from build123d import *

# Parameters (mm, degrees)
F2_DEPTH = 1.2
F3_DEPTH = 2.4
F4_R     = 2
F5_R     = 1
F6_SIZE  = 0.4


with BuildPart() as f2:
    # F1 (on Top) → F2 (new body)
    with BuildSketch(Plane.XY):
        Polygon((-15.6, 7.5), (-15.6, 5.7), (-0.9, 0), (-15.6, -5.7), (-15.6, -7.5), (-0.6, -7.5), (-0.6, 0), (-0.6, 7.5), align=None)
    extrude(amount=F2_DEPTH)



with BuildPart() as f2b:
    # F1 (on Top) → F2, piece 2 (new body)
    with BuildSketch(Plane.XY):
        Polygon((0.9, 0), (15.6, 5.7), (15.6, 7.5), (0.6, 7.5), (0.6, 0), (0.6, -7.5), (15.6, -7.5), (15.6, -5.7), align=None)
    extrude(amount=F2_DEPTH)


with BuildPart() as f2_1:
    add(f2.part)

    add(f2b.part)  # F3 merges F2b
    # F1 (on Top) → F3 (join)
    with BuildSketch(Plane.XY):
        Polygon((0, 8.7), (-16.8, 8.7), (-16.8, 5.7), (-15.6, 5.7), (-15.6, 7.5), (-0.6, 7.5), (-0.6, 0), (-0.6, -7.5), (-15.6, -7.5), (-15.6, -5.7), (-16.8, -5.7), (-16.8, -8.7), (0, -8.7), (16.8, -8.7), (16.8, -5.7), (15.6, -5.7), (15.6, -7.5), (0.6, -7.5), (0.6, 0), (0.6, 7.5), (15.6, 7.5), (15.6, 5.7), (16.8, 5.7), (16.8, 8.7), align=None)
    extrude(amount=F3_DEPTH)

    # F4
    f4_edges = [f2_1.edges().sort_by_distance(p)[0] for p in [
        (-0.9, 0, 0.6),
        (0.9, 0, 0.6),
    ]]
    fillet(f4_edges, radius=F4_R)

    # F5
    f5_edges = [f2_1.edges().sort_by_distance(p)[0] for p in [
        (16.8, -8.7, 1.2),
        (16.8, 8.7, 1.2),
        (-16.8, -8.7, 1.2),
        (-16.8, 8.7, 1.2),
    ]]
    fillet(f5_edges, radius=F5_R)

    # F6
    f6_edges = [f2_1.edges().sort_by_distance(p)[0] for p in [
        (16.8, 6.7, 0),
        (16.507107, 8.407107, 0),
        (16.2, 5.7, 0),
        (0, 8.7, 0),
        (10.654511, 3.782361, 0),
        (-16.507107, 8.407107, 0),
        (4.432077, 0, 0),
        (-16.8, 6.7, 0),
        (10.654511, -3.782361, 0),
        (-16.2, 5.7, 0),
        (16.2, -5.7, 0),
        (-10.654511, 3.782361, 0),
        (16.8, -6.7, 0),
        (-4.432077, 0, 0),
        (16.507107, -8.407107, 0),
        (-10.654511, -3.782361, 0),
        (0, -8.7, 0),
        (-16.2, -5.7, 0),
        (-16.507107, -8.407107, 0),
        (-16.8, -6.7, 0),
        (-10.654511, -3.782361, 1.2),
        (4.432077, 0, 1.2),
    ]]
    chamfer(f6_edges, length=F6_SIZE)


solid = f2_1.part
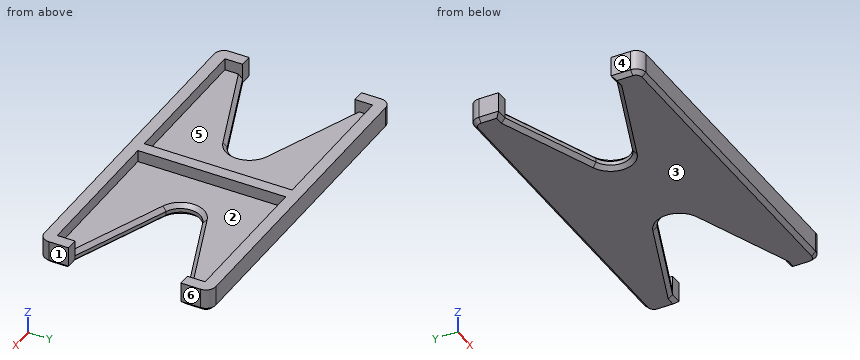
Read the model definition and answer for the solid it produces. Units are mm, in the model's axes. Face numbers are marked on the shaded views. A direction names the side the tool comes from. Coordinates: 2 decimals unless noted, no trailing zeros. Loops run counter-clockwise (first coordinate to the right, second up) from the corner with the lowest first, then second, coordinate; pieces in that order, holes last.
Q1. The part is cut by section C-C on x = 1.5. Write down the section's boundary in (y, z).
Q2. Consider probe 1 along Y at (x, z) = (10, 1.75); probe 2 along Z at (x, y) = (-3, -5.75); probe 3 along X at (y, z) = (5.25, 1.3). Determine where each line is inside the solid, lowest interval first.
Q3. The part is cut by section D-D on z = 1.8. Write down the section's boundary in (x, y).
Q4. This flat-tipped pin is pushed along its axis until it touches: pin 1 Ø1.3 at (y, z) = (1, 1.5) entering from +X. Where does it stop, or does it pass through?
Q5. The part is cut by section B-B on y = 7. Write down the section's boundary in (x, z), and give its area (3 significant figures).
Q6. The mould has two halves that part along X. Classify the marked faces 3, 4, 5 and 6: +X half, -X half, draft (parallel to the pull), parting line (faces both ways), or undercut.
Q7. Which of the six approach directions +Z, -Z, +X, -X, +Y, -Y give full straight-line access (tool end or side, diameter ignored) to the marked faces 1 and 2?
Q8. The part is cut by section A-A on x = -9.5. Write down the section's boundary in (y, z), and give its area (3 significant figures).
Results below:
1. outline: (-8.7, 0.4) - (-8.3, 0) - (8.3, 0) - (8.7, 0.4) - (8.7, 2.4) - (7.5, 2.4) - (7.5, 1.2) - (-7.5, 1.2) - (-7.5, 2.4) - (-8.7, 2.4) - close
2. probe 1: y = -8.7 to -7.5, 7.5 to 8.7
2. probe 2: z = 0 to 1.2
2. probe 3: x = -0.6 to 0.6
3. outline: (-16.8, -7.7) arc R1 ccw to (-15.8, -8.7) - (15.8, -8.7) arc R1 ccw to (16.8, -7.7) - (16.8, -5.7) - (15.6, -5.7) - (15.6, -7.5) - (0.6, -7.5) - (0.6, 7.5) - (15.6, 7.5) - (15.6, 5.7) - (16.8, 5.7) - (16.8, 7.7) arc R1 ccw to (15.8, 8.7) - (-15.8, 8.7) arc R1 ccw to (-16.8, 7.7) - (-16.8, 5.7) - (-15.6, 5.7) - (-15.6, 7.5) - (-0.6, 7.5) - (-0.6, -7.5) - (-15.6, -7.5) - (-15.6, -5.7) - (-16.8, -5.7) - close
4. pin 1: stops at x = 4.76
5. outline: (-16.8, 0.4) - (-16.4, 0) - (16.4, 0) - (16.8, 0.4) - (16.8, 2.4) - (15.6, 2.4) - (15.6, 1.2) - (0.6, 1.2) - (0.6, 2.4) - (-0.6, 2.4) - (-0.6, 1.2) - (-15.6, 1.2) - (-15.6, 2.4) - (-16.8, 2.4) - close
5. area: 44.5 mm2
6. face 3: draft
6. face 4: -X half
6. face 5: undercut
6. face 6: +X half
7. face 1: +Z, -Z, +X, +Y, -Y
7. face 2: +Z
8. outline: (-8.7, 0.4) - (-8.3, 0) - (-3.76, 0) - (-3.33, 0.4) - (-3.33, 0.8) - (-3.76, 1.2) - (-7.5, 1.2) - (-7.5, 2.4) - (-8.7, 2.4) - close; (3.33, 0.4) - (3.76, 0) - (8.3, 0) - (8.7, 0.4) - (8.7, 2.4) - (7.5, 2.4) - (7.5, 1.2) - (3.76, 1.2) - (3.33, 0.8) - close
8. area: 15.3 mm2
